Build history of the part. All positions in model axes, mm. Round coordinates to 2 decimals unless told otherwise and drop trailing zeros. Write each loop counter-clockwise with the first axis right and the second up, starting at its lowest first coordinate (ties: lowest second). Pieces come first, ordered by that corner, then holes.
Item 1: Band-saw the part on A-A, the plane z = -8.5. Write the cut outline in (x, y), then the cut area to 3 significant figures.
Item 2: Drop a flat-ended pin along its axis: pin 1 Ø6.5 at (x, z) = (855.5, -7.5) entering from +Y. Give the stop position or say it passes through.
Item 3: Wall check: probe 1 along X at (y, z) = (33.5, -7.75); probe 2 along Y at (x, z) = (436, -6.5). Give the ranges that are in metal, low to high.
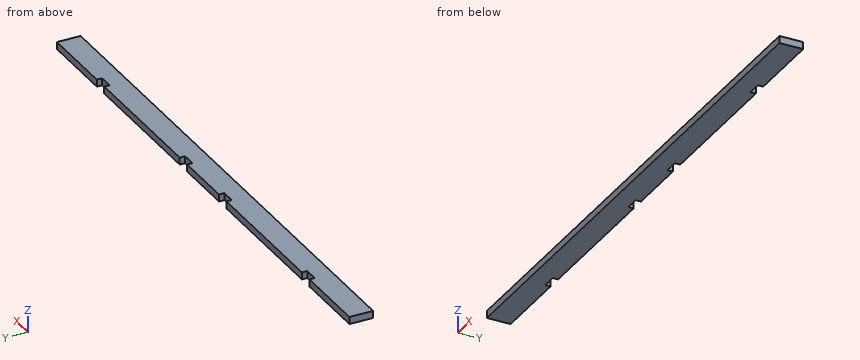
Autodesk Inventor part; units mm, degrees
ref_plane "YZ Plane" through (0, 0, 0) normal (1, 0, 0) x (0, 1, 0)
ref_plane "XZ Plane" through (0, 0, 0) normal (0, 1, 0) x (-1, 0, 0)
ref_plane "XY Plane" through (0, 0, 0) normal (0, 0, 1) x (1, 0, 0)
sketch "Sketch1" plane through (0, 0, 0) normal (0, 0, 1) x (1, 0, 0)
  line L0 (0, 0) -> (1003.3, 0)
  line L1 (1003.3, 0) -> (1003.3, 42.3672)
  line L2 (1003.3, 42.3672) -> (0, 42.3672)
  line L3 (0, 42.3672) -> (0, 0)
  dimension "d0" = 42.3672
  dimension "d1" = 1003.3
extrude "Extrusion1" add sketch "Sketch1" against normal blind 12.7
sketch "Sketch2" plane through (0, 0, 0) normal (0, 0, 1) x (1, 0, 0)
  line L0 (1003.3, 0) -> (1003.3, 42.3672)
  line L1 (1003.3, 42.3672) -> (0, 42.3672)
  line L2 (0, 42.3672) -> (0, 0)
  line L3 (137.16, 42.3672) -> (162.56, 42.3672)
  line L4 (162.56, 42.3672) -> (162.56, 32.8422)
  line L5 (162.56, 32.8422) -> (137.16, 32.8422)
  line L6 (137.16, 32.8422) -> (137.16, 42.3672)
  line L7 (866.14, 42.3672) -> (840.74, 42.3672)
  line L8 (840.74, 42.3672) -> (840.74, 32.8422)
  line L9 (840.74, 32.8422) -> (866.14, 32.8422)
  line L10 (866.14, 32.8422) -> (866.14, 42.3672)
  line L11 (421.64, 42.3672) -> (447.04, 42.3672)
  line L12 (447.04, 42.3672) -> (447.04, 32.8422)
  line L13 (447.04, 32.8422) -> (421.64, 32.8422)
  line L14 (421.64, 32.8422) -> (421.64, 42.3672)
  line L15 (581.66, 42.3672) -> (556.26, 42.3672)
  line L16 (556.26, 42.3672) -> (556.26, 32.8422)
  line L17 (556.26, 32.8422) -> (581.66, 32.8422)
  line L18 (581.66, 32.8422) -> (581.66, 42.3672)
  dimension "d4" = 9.525
  dimension "d5" = 25.4
  dimension "d6" = 137.16
  dimension "d7" = 137.16
  dimension "d8" = 25.4
  dimension "d9" = 9.525
  dimension "d12" = 421.64
  dimension "d13" = 25.4
  dimension "d14" = 9.525
  dimension "d15" = 421.64
  dimension "d16" = 25.4
  dimension "d17" = 9.525
extrude "Extrusion3" cut sketch "Sketch2" against normal blind 12.7
properties part number "spacer 2"
Results:
1. outline: (0, 0) - (1003.3, 0) - (1003.3, 42.37) - (866.14, 42.37) - (866.14, 32.84) - (840.74, 32.84) - (840.74, 42.37) - (581.66, 42.37) - (581.66, 32.84) - (556.26, 32.84) - (556.26, 42.37) - (447.04, 42.37) - (447.04, 32.84) - (421.64, 32.84) - (421.64, 42.37) - (162.56, 42.37) - (162.56, 32.84) - (137.16, 32.84) - (137.16, 42.37) - (0, 42.37) - close
1. area: 41,500 mm2
2. pin 1: stops at y = 32.84
3. probe 1: x = 0 to 137.16, 162.56 to 421.64, 447.04 to 556.26, 581.66 to 840.74, 866.14 to 1003.3
3. probe 2: y = 0 to 32.84
